Could you check a few things on this model? Use its own coordinates, in mm. Face numbers are marked on the shaded views. A direction names the side the tool comes from. Round coordinates to 2 decimals unless told otherwise and drop trailing zeros. Loops run counter-clockwise (first coordinate to the right, second up) from the corner with the lowest first, then second, coordinate; pieces in that order, holes last. Notation, with made-up numbers: (-32, 87) -> (-7, 87) arc R17 ccw to (-7, 106) -> close; hole circle Ø2 at (74.5, 73). An arc over 180 degrees is marked (long way). One line per item, written item: value.
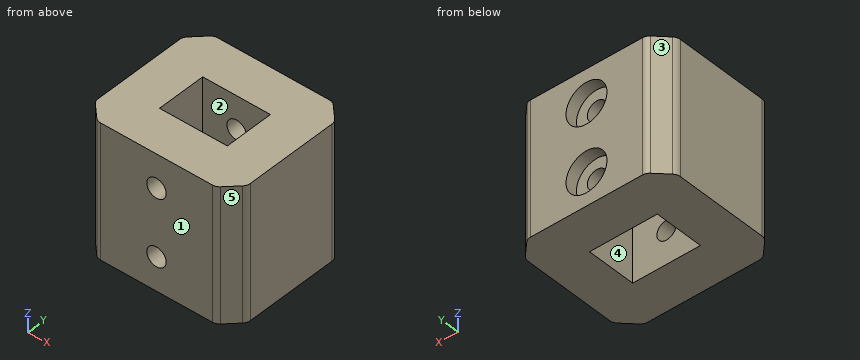
```python
from build123d import *

# Parameters (mm, degrees)
SKETCH1_W                               = 45.5
SKETCH1_H                               = 40
SKETCH1_W_2                             = 20.25
SKETCH1_H_2                             = 14.75
BOSS_EXTRUDE1_DEPTH                     = 40
CHAMFER1_SIZE                           = 5
FILLET1_R                               = 2.5
CBORE_FOR_M5_HEX_HEAD_BOLT1_D           = 5.8
CBORE_FOR_M5_HEX_HEAD_BOLT1_CBORE_D     = 12.24
CBORE_FOR_M5_HEX_HEAD_BOLT1_CBORE_DEPTH = 3.58


with BuildPart() as part:
    # Sketch1 → Boss-Extrude1 (new body)
    with BuildSketch(Plane.XY):
        Rectangle(SKETCH1_W, SKETCH1_H)
        Rectangle(SKETCH1_W_2, SKETCH1_H_2, mode=Mode.SUBTRACT)
    extrude(amount=BOSS_EXTRUDE1_DEPTH)

    # Chamfer1
    chamfer1_edges = [part.edges().sort_by_distance(p)[0] for p in [
        (22.75, -20, 20),
        (-22.75, -20, 20),
        (-22.75, 20, 20),
        (22.75, 20, 20),
    ]]
    chamfer(chamfer1_edges, length=CHAMFER1_SIZE)

    # Fillet1
    fillet1_edges = [part.edges().sort_by_distance(p)[0] for p in [
        (-17.75, 20, 20),
        (17.75, 20, 20),
        (22.75, -15, 20),
        (22.75, 15, 20),
        (-17.75, -20, 20),
        (17.75, -20, 20),
        (-22.75, 15, 20),
        (-22.75, -15, 20),
    ]]
    fillet(fillet1_edges, radius=FILLET1_R)

    # CBORE for M5 Hex Head Bolt1 (through all)
    with Locations(Plane(origin=(0, 20, 0), x_dir=(1, 0, 0), z_dir=(0, 1, 0))):
        with Locations((0, -10)):
            cbore_for_m5_hex_head_bolt1 = CounterBoreHole(CBORE_FOR_M5_HEX_HEAD_BOLT1_D / 2, CBORE_FOR_M5_HEX_HEAD_BOLT1_CBORE_D / 2, CBORE_FOR_M5_HEX_HEAD_BOLT1_CBORE_DEPTH)

    # Mirror1: CBORE for M5 Hex Head Bolt1 across plane
    add(cbore_for_m5_hex_head_bolt1.mirror(Plane(origin=(0, 0, 20), x_dir=(1, 0, 0), z_dir=(0, 0, -1))), mode=Mode.SUBTRACT)


solid = part.part
```
(1) Imagine slicing it at B-B on y = -4. Write out the boundary of the cut face in (x, z) (3 decimals).
Results below:
outline: (-22.75, 0) -> (-10.125, 0) -> (-10.125, 40) -> (-22.75, 40) -> close; (10.125, 0) -> (22.75, 0) -> (22.75, 40) -> (10.125, 40) -> close
(2) Imagine slicing it at A-A on x = 8. Write out the boundary of the cut face in (y, z) (3 decimals).
Results below:
outline: (-20, 0) -> (-7.375, 0) -> (-7.375, 40) -> (-20, 40) -> close; (7.375, 0) -> (20, 0) -> (20, 40) -> (7.375, 40) -> close
(3) For pin 1 Ø3.5 at (x, z) = (-1, 7.5) entering from +Y, with a flat end and sliding along its axis, tell me the tip position at first contact or that it passes through.
Results below:
pin 1: stops at y = 16.42
(4) Please list where these lines run through material, in increasing order: L1, parallel to Z at x = 0, y = 13; L2, parallel to Z at x = 0, y = 18.8; L3, parallel to Y at x = -1, z = 24.5 (3 decimals).
Results below:
L1: z = 0 to 7.1, 12.9 to 27.1, 32.9 to 40
L2: z = 0 to 3.88, 16.12 to 23.88, 36.12 to 40
L3: y = -20 to -7.375, 7.375 to 16.42
(5) Imagine slicing it at C-C on x = 0. Give the number of separate pieces and of enclosed holes in the cut face, then the cut area to 3 significant figures.
Results below:
separate pieces: 6
enclosed holes: 0
area: 671 mm²
(6) On a 3-axis mill with a long thin cutter (end or side, diameter ignored), from which of +Z, -Z, +X, -X, +Y, -Y can I reach the whole of each face in a straight line? I mean the marked faces 1 and 2. Say none if no direction works.
Results below:
face 1: +Z, -Z, +X, -X, -Y
face 2: +Z, -Z
(7) We'd pull the mould along X, two halves only. Please class the marked faces 3, 4 and 5: +X half, -X half, draft (parallel to the pull), parting line (faces both ways), or undercut.
Results below:
face 3: -X half
face 4: undercut
face 5: +X half
